from build123d import *

# Parameters (mm, degrees)
F0_R     = 22.5
F0_R_2   = 10
F1_DEPTH = 6
F2_R     = 13.65
F2_R_2   = 10
F3_DEPTH = 3
F4_R     = 19.5
F4_R_2   = 11.5
F5_DEPTH = 4


with BuildPart() as f1:
    # F0 (on Top) → F1 (new body)
    with BuildSketch(Plane.XY):
        Circle(F0_R)
        Circle(F0_R_2, mode=Mode.SUBTRACT)
    extrude(amount=F1_DEPTH)

    # F2 (on face) → F3 (join)
    with BuildSketch(Plane.XY.offset(6)):
        Circle(F2_R)
        Circle(F2_R_2, mode=Mode.SUBTRACT)
    extrude(amount=F3_DEPTH)

    # F4 (on face) → F5 (cut)
    with BuildSketch(Plane.XY):
        Circle(F4_R)
        Circle(F4_R_2, mode=Mode.SUBTRACT)
    extrude(amount=F5_DEPTH, mode=Mode.SUBTRACT)


solid = f1.part
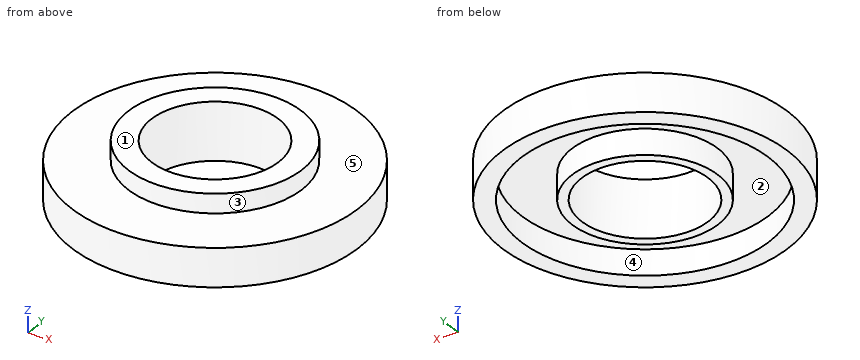
Work out the finished part from the listing and answer in its coordinate system (mm). Face numbers are marked on the shaded views. A direction names the side the tool comes from. Round coordinates to 2 decimals unless told otherwise and drop trailing zeros. Order: outer loops, then holes, each group sorted by start corner. A loop starts at its lowest first (then second) coordinate and runs counter-clockwise, first axis right, second up. Notation, with made-up numbers: M 13,22.5 L 49,22.5 A33 cw 49,57.5 Z; hole C 63.25,-2.5 d3. An arc over 180 degrees is marked long. Put each result on its own line as item: value. Start each with the question number.
Q1. Flat-ended cylindrical pins translate along their axes: pin 1 (2 mm diameter, centred on x = -13, z = 2.5, fed in from -Y); pin 2 (4 mm diameter, centred on x = 8, z = 6.5, fed in from -Y); pin 3 (4 mm diameter, centred on y = -12, z = 3, fed in from -X); pin 4 (4 mm diameter, centred on x = -16, y = 9, fed in from -Z). Find the tip coordinate at first contact, or state that the pin passes through.
Q2. Straight lines are drawn through the part: L1, parallel to Y at x = 0, z = 2.4; L2, parallel to Y at x = 0, z = 6.25; L3, parallel to X at y = 0.5, z = 0.5. For each, find the intervals that lie inside material, in ascending order. Write a range as [from, to].
Q3. Section C-C, the plane z = 1 is taken. Write down the section's boundary in (x, y), and give its area (3 significant figures).
Q4. For a pull along X with two mould halves and no side action, classify the marked faces 3, 4 and 5 as pulls with the +X half, pulls with the -X half, needs draft (parallel to the pull), parting line crosses it, or undercut.
Q5. Section D-D, the plane z = 5 is taken. Write down the section's boundary in (x, y), and give its area (3 significant figures).
Q6. Section A-A, the plane x = 0 is taken. Write down the section's boundary in (y, z).
Q7. A tool of negligible diameter and unlimited length cuts with its end or side. For the marked faces 1 and 2, from which of +Z, -Z, +X, -X, +Y, -Y can it reach the whole face along a straight path? Write none if from no direction.
Findings below:
1. pin 1: stops at y = -19.03
1. pin 2: stops at y = -21.67
1. pin 3: stops at x = -20.16
1. pin 4: stops at z = 0
2. L1: y = [-22.5, -19.5], [-11.5, -10], [10, 11.5], [19.5, 22.5]
2. L2: y = [-13.65, -10], [10, 13.65]
2. L3: x = [-22.49, -19.49], [-11.49, -9.99], [9.99, 11.49], [19.49, 22.49]
3. outline: C 0,0 d45; C 0,0 d23; hole C 0,0 d39; hole C 0,0 d20
3. area: 497 mm^2
4. face 3: parting line crosses it
4. face 4: undercut
4. face 5: needs draft
5. outline: C 0,0 d45; hole C 0,0 d20
5. area: 1,280 mm^2
6. outline: M -22.5,0 L -19.5,0 L -19.5,4 L -11.5,4 L -11.5,0 L -10,0 L -10,9 L -13.65,9 L -13.65,6 L -22.5,6 Z; M 10,0 L 11.5,0 L 11.5,4 L 19.5,4 L 19.5,0 L 22.5,0 L 22.5,6 L 13.65,6 L 13.65,9 L 10,9 Z
7. face 1: +Z, +X, -X, +Y, -Y
7. face 2: -Z
